from build123d import *

# Parameters (mm, degrees)
F1_DEPTH = 2
F3_DEPTH = 2


with BuildPart() as f1:
    # F0 (on Front) → F1 (new body)
    with BuildSketch(Plane.XZ):
        Polygon((3.9369898587, 45), (0, 0), (17, 0), (17, 10), (19, 10), (19, 2), (33.5, 2), (33.5, 10), (35.5, 10), (35.5, 2), (50, 2), (50, 10), (52, 10), (52, 2), (66.5, 2), (66.5, 10), (68.5, 10), (68.5, 2), (83, 2), (83, 10), (85, 10), (85, 2), (99.5, 2), (99.5, 10), (101.5, 10), (101.5, 2), (116, 2), (116, 10), (118, 10), (118, 2), (132.5, 2), (132.5, 10), (134.5, 10), (134.5, 2), (149, 2), (149, 10), (151, 10), (151, 2), (165.5, 2), (165.5, 10), (167.5, 10), (167.5, 2), (182, 2), (182, 10), (184, 10), (184, 2), (198.5, 2), (198.5, 10), (200.5, 10), (200.5, 2), (215, 2), (215, 10), (217, 10), (217, 2), (231.5, 2), (231.5, 10), (233.5, 10), (233.5, 2), (248, 2), (248, 10), (250, 10), (250, 2), (264.5, 2), (264.5, 10), (266.5, 10), (266.5, 2), (281, 2), (281, 10), (283, 10), (283, 0), (300, 0), (296.0630101413, 45), (291.0630101413, 45), (290.6255668237, 50), (283, 50), (283, 35), (281, 35), (281, 50), (266.5, 50), (266.5, 35), (264.5, 35), (264.5, 50), (250, 50), (250, 35), (248, 35), (248, 50), (233.5, 50), (233.5, 35), (231.5, 35), (231.5, 50), (217, 50), (217, 35), (215, 35), (215, 50), (200.5, 50), (200.5, 35), (198.5, 35), (198.5, 50), (184, 50), (184, 35), (182, 35), (182, 50), (167.5, 50), (167.5, 35), (165.5, 35), (165.5, 50), (151, 50), (151, 35), (149, 35), (149, 50), (134.5, 50), (134.5, 35), (132.5, 35), (132.5, 50), (118, 50), (118, 35), (116, 35), (116, 50), (101.5, 50), (101.5, 35), (99.5, 35), (99.5, 50), (85, 50), (85, 35), (83, 35), (83, 50), (68.5, 50), (68.5, 35), (66.5, 35), (66.5, 50), (52, 50), (52, 35), (50, 35), (50, 50), (35.5, 50), (35.5, 35), (33.5, 35), (33.5, 50), (19, 50), (19, 35), (17, 35), (17, 50), (9.3744331763, 50), (8.9369898587, 45), align=None)
    extrude(amount=-F1_DEPTH)

    # F2 (on Front) → F3 (cut, through all)
    with BuildSketch(Plane.XZ):
        Polygon((283, 20), (17, 20), (17, 16), (24, 16), (24, 15), (27.7, 15), (27.7, 16), (40.5, 16), (40.5, 15), (44.2, 15), (44.2, 16), (57, 16), (57, 15), (60.7, 15), (60.7, 16), (73.5, 16), (73.5, 15), (77.2, 15), (77.2, 16), (90, 16), (90, 15), (93.7, 15), (93.7, 16), (106.5, 16), (106.5, 15), (110.2, 15), (110.2, 16), (123, 16), (123, 15), (126.7, 15), (126.7, 16), (139.5, 16), (139.5, 15), (143.2, 15), (143.2, 16), (156, 16), (156, 15), (159.7, 15), (159.7, 16), (172.5, 16), (172.5, 15), (176.2, 15), (176.2, 16), (189, 16), (189, 15), (192.7, 15), (192.7, 16), (205.5, 16), (205.5, 15), (209.2, 15), (209.2, 16), (222, 16), (222, 15), (225.7, 15), (225.7, 16), (238.5, 16), (238.5, 15), (242.2, 15), (242.2, 16), (255, 16), (255, 15), (258.7, 15), (258.7, 16), (271.5, 16), (271.5, 15), (275.2, 15), (275.2, 16), (283, 16), align=None)
        Polygon((1.3123299529, 15), (0.4374433176, 5), (5.4374433176, 5), (6.3123299529, 15), align=None)
        Polygon((298.6876700471, 15), (293.6876700471, 15), (294.5625566824, 5), (299.5625566824, 5), align=None)
    extrude(amount=-F3_DEPTH, mode=Mode.SUBTRACT)


solid = f1.part
Geometry: final body of the model. Coordinates: model frame, mm. Give positions to 0.01 mm unless a question says otherwise; leave off trailing zeros. Answer in a Markdown table with one row per item.
(1) Ray query, line 1 along Z through (x, y) = (155.5, 1.6); line 2 along Z through (x, y) = (90.5, 0.75); line 3 along X through (y, z) = (1.1, 23). Return the intervals inside material, ascending. Write a range as [from, to].
Answers below:
| item | result |
|---|---|
| line 1 | [2, 16], [20, 50] |
| line 2 | [2, 15], [20, 50] |
| line 3 | [2.01, 297.99] |
(2) Draft query along Y for faces 1 (the flat face through (148, 0, 25)), 2 (the flat face through (148, 2, 25)). Return one class per face: +Y half, -Y half, draft (parallel to the pull), parting line (faces both ways), or undercut.
Answers below:
| item | result |
|---|---|
| face 1 | -Y half |
| face 2 | +Y half |
(3) Pin query (flat end, axial travel): pin 1 (1 mm diameter, centred on x = 44, y = 1, fed in from -Z); pin 2 (0.6 mm diameter, centred on y = 1.5, z = 42.5, fed in from -X); pin 3 (1 mm diameter, centred on y = 1.5, z = 36, fed in from +X). Return the tip coordinate at first contact, or that it passes through.
Answers below:
| item | result |
|---|---|
| pin 1 | z = 2 |
| pin 2 | x = 3.69 |
| pin 3 | x = 296.89 |
